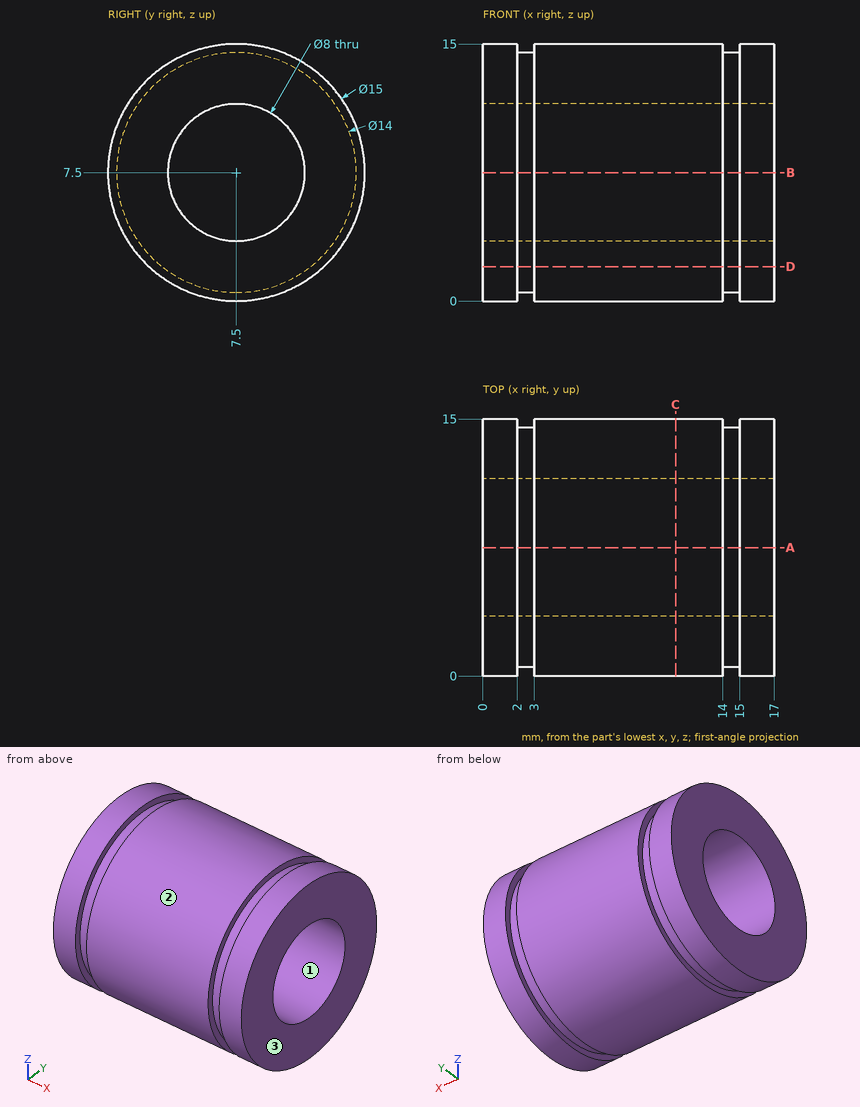
Source: three-view drawing plus pictorial views. Frame: mm from the lowest corner of the part. Round coordinates to 2 decimals unless told otherwise and drop trailing zeros. Loops run counter-clockwise (first coordinate to the right, second up) from the corner with the lowest first, then second, coordinate; pieces in that order, holes last.
Q1. Section D-D, the plane z = 2. Return loops of the section in (x, y).
Q2. First-contact query: P1, Ø5, axis at y = 7.5, z = 7.5, coming from the -X side; P2, Ø6, axis at x = 10, z = 2, coming from the +Y side; P3, Ø4, axis at x = 10, z = 10.5, coming from the +Y side; P4, Ø2, axis at x = 10, z = 3.5, coming from the +Y side. Flat tips, straight axial feed; report the tip coordinate or a pass-through.
Q3. Ray query, line 1 (Y direction, x = 10, z = 7.5); line 2 (Z direction, x = 16, y = 5.5); line 3 (Y direction, x = 11.5, z = 4.25). Return the intervals inside material, ascending.
Q4. Mould query, pull axis Z, two halves, no side actions, for the marked faces 1, 2 and 3. Classes: pulls with the +Z half, pulls with the -Z half, needs draft (parallel to the pull), parting line crosses it, or undercut.
Q5. Section A-A, the plane y = 7.5. Return loops of the section in (x, z), plus the area to 3 significant figures.
Q6. Section C-C, the plane x = 11.25. Return loops of the section in (y, z).
Solutions:
1. outline: (0, 2.4) - (2, 2.4) - (2, 3.17) - (3, 3.17) - (3, 2.4) - (14, 2.4) - (14, 3.17) - (15, 3.17) - (15, 2.4) - (17, 2.4) - (17, 12.6) - (15, 12.6) - (15, 11.83) - (14, 11.83) - (14, 12.6) - (3, 12.6) - (3, 11.83) - (2, 11.83) - (2, 12.6) - (0, 12.6) - close
2. P1: passes through
2. P2: stops at y = 14.57
2. P3: stops at y = 14.93
2. P4: stops at y = 14.37
3. line 1: y = 0 to 3.5, 11.5 to 15
3. line 2: z = 0.27 to 4.04, 10.96 to 14.73
3. line 3: y = 0.74 to 5.17, 9.83 to 14.26
4. face 1: undercut
4. face 2: parting line crosses it
4. face 3: needs draft
5. outline: (0, 0) - (2, 0) - (2, 0.5) - (3, 0.5) - (3, 0) - (14, 0) - (14, 0.5) - (15, 0.5) - (15, 0) - (17, 0) - (17, 3.5) - (0, 3.5) - close; (0, 11.5) - (17, 11.5) - (17, 15) - (15, 15) - (15, 14.5) - (14, 14.5) - (14, 15) - (3, 15) - (3, 14.5) - (2, 14.5) - (2, 15) - (0, 15) - close
5. area: 117 mm2
6. outline: circle Ø15 at (7.5, 7.5); hole circle Ø8 at (7.5, 7.5)
